Check sheet for the drawn part. Datum: minimum x, y, z corner. Units: mm. Round coordinates to 2 decimals unless told otherwise and drop trailing zeros. Write each loop counter-clockwise with the first axis right and the second up, starting at its lowest first coordinate (ties: lowest second). Pieces come first, ordered by that corner, then holes. Notation, with made-up numbers: M -39.5,11.25 L 8.5,11.25 A17 cw 8.5,16.25 Z; hole C 78,32 d3. An arc over 180 degrees is marked long. One line per item, written item: value. Start each with the question number.
Item 1: Section check A-A, the plane x = 30. Record the cut outline in (y, z).
Item 2: Section check C-C, the plane y = 32. Record the cut outline in (x, z).
Item 3: Thickness scan on probe 1 along X at (y, z) = (48.05, 80.5); probe 2 along Z at (x, y) = (30, 49); probe 3 along X at (y, z) = (49, 80). Record the ranges inside material, lowest first. Write a range as from..to.
Item 4: Gauge pin test, flat ends, axial feed: pin 1 (17 mm diameter, centred on x = 35, z = 29, fed in from -Y); pin 2 (3.5 mm diameter, centred on x = 2, z = 63.5, fed in from -Y). Record the tip position at first contact, or that the pin passes through.
Item 5: Section check B-B, the plane z = 49. Record the cut outline in (x, y).
Item 6: Draft check along Y on the marked faces 1, 2 and 3. Enter one of: +Y half, -Y half, draft (parallel to the pull), parting line (faces both ways), or undercut.
Item 7: Section check D-D, the plane z = 65.5. Record the cut outline in (x, y), then the cut area to 3 significant figures.
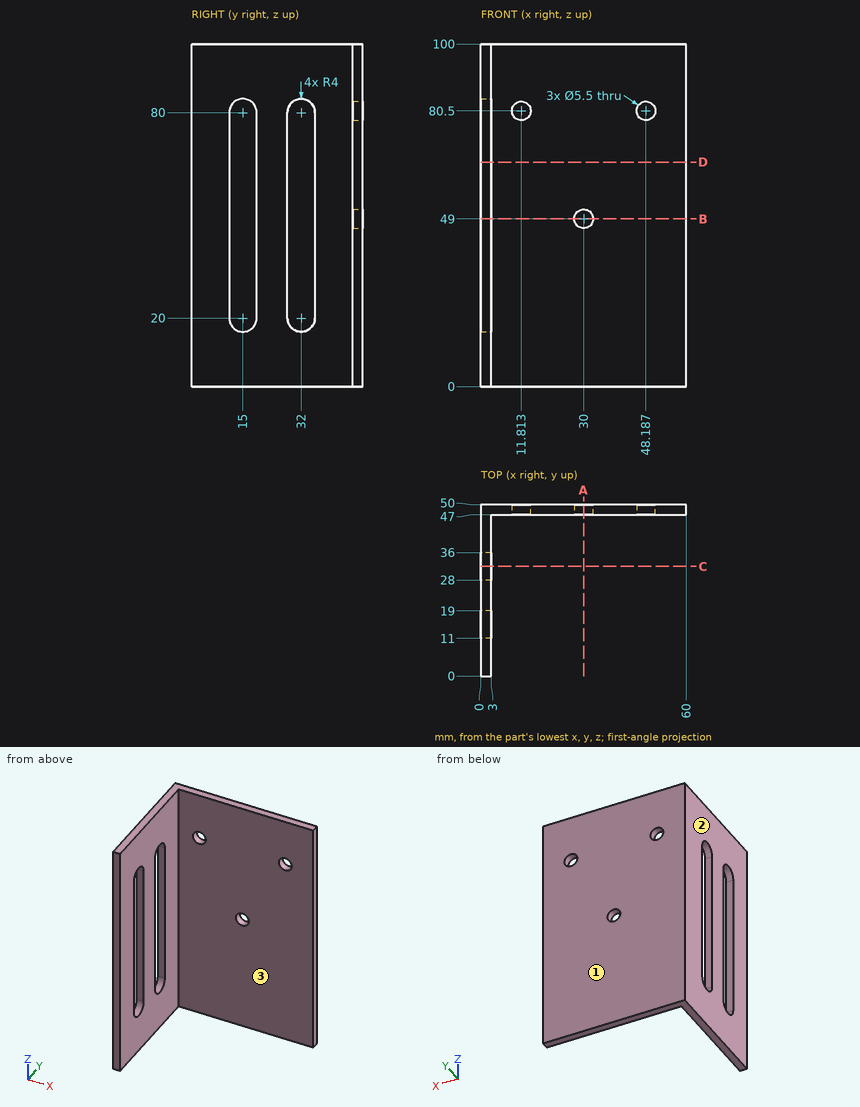
Response values:
1. outline: M 47,0 L 50,0 L 50,46.25 L 47,46.25 Z; M 47,51.75 L 50,51.75 L 50,100 L 47,100 Z
2. outline: M 0,0 L 3,0 L 3,16 L 0,16 Z; M 0,84 L 3,84 L 3,100 L 0,100 Z
3. probe 1: x = 0..9.06, 14.56..45.44, 50.94..60
3. probe 2: z = 0..46.25, 51.75..100
3. probe 3: x = 0..9.11, 14.52..45.48, 50.89..60
4. pin 1: stops at y = 47
4. pin 2: stops at y = 0
5. outline: M 0,0 L 3,0 L 3,11 L 0,11 Z; M 0,19 L 3,19 L 3,28 L 0,28 Z; M 0,36 L 3,36 L 3,47 L 27.25,47 L 27.25,50 L 0,50 Z; M 32.75,47 L 60,47 L 60,50 L 32.75,50 Z
6. face 1: +Y half
6. face 2: draft
6. face 3: -Y half
7. outline: M 0,0 L 3,0 L 3,11 L 0,11 Z; M 0,19 L 3,19 L 3,28 L 0,28 Z; M 0,36 L 3,36 L 3,47 L 60,47 L 60,50 L 0,50 Z
7. area: 273 mm2
